CAD build for the part. Positions are in the model's coordinates, mm. A direction names the side the tool comes from. Coordinates: 2 decimals unless noted, no trailing zeros. Loops run counter-clockwise (first coordinate to the right, second up) from the corner with the lowest first, then second, coordinate; pieces in that order, holes last. Notation, with made-up numbers: (18.25, 20.25) -> (38.25, 20.25) arc R9 cw to (38.25, 36.25) -> close; hole circle Ø3 at (-31.75, 19.5). An arc over 180 degrees is marked (long way). Write each question's results on one line, items separated by ' | '.
Autodesk Inventor part; units mm, degrees
ref_plane "YZ Plane" through (0, 0, 0) normal (1, 0, 0) x (0, 1, 0)
ref_plane "XZ Plane" through (0, 0, 0) normal (0, 1, 0) x (-1, 0, 0)
ref_plane "XY Plane" through (0, 0, 0) normal (0, 0, 1) x (1, 0, 0)
sketch "Sketch1" plane through (0, 0, 0) normal (0, 1, 0) x (-1, 0, 0)
  line L0 (0, 44.45) -> (-22.5, 44.45)
  line L1 (-22.5, 44.45) -> (-67.5, 24.15)
  line L2 (-67.5, 24.15) -> (-90, 24.15)
  line L3 (-90, 0) -> (0, 0)
  line L4 (-90, 22.15) -> (-66.3402, 22.15)
  line L5 (-66.3402, 22.15) -> (-22.0052, 42.15)
  line L6 (-22.0052, 42.15) -> (0, 42.15)
  line L7 (-90, 0) -> (-90, 22.15) construction
  line L8 (-90, 24.15) -> (-90, 22.15)
  line L9 (0, 44.45) -> (0, 42.15)
  line L10 (0, 0) -> (0, 42.15) construction
  line L11 (-45, 34.3) -> (-44.0542, 32.2035) construction
  dimension "d0" = 88.9
  dimension "d1" = 48.3
  dimension "d2" = 2.3
  dimension "d3" = 2
  dimension "d4" = 90
  dimension "d5" = 22.5
  dimension "d6" = 22.5
  dimension "d10" = 2.3
revolve "Revolution1" add sketch "Sketch1" angle 360 about axis through (90, 0, 0) along (-1, 0, 0)
equation "\"d0\" = D1"
equation "\"d1\" = D2"
equation "\"d2\" = s1"
equation "\"d3\" = s2"
equation "\"d4\" = L"
equation "\"d5\" = 0.25 * L"
equation "\"d6\" = 0.25 * L"
equation "\"d10\" = s3"
equation "\"s1\" = 2.3"
equation "\"D1\" = 88.9"
equation "\"D2\" = 48.3"
equation "\"L\" = 90"
equation "\"s2\" = 2"
equation "\"s3\" = 2.3"
equation "\"Size_Designation\" = 1.2345"
properties part number "DIN 2616 Concentric Reducer (K) 88.9 x 2.3 - 48.3 x 2" material "Steel"
Q1. Pull direction Z, two halves, no side cores. Call faces 3 (the flat face through (90, -20, 11)), 4 (the cylindrical face through (78.908, -1.062, -24.127)), 5 (the cylindrical face through (78.004, -21.623, -4.802)): +Z half, -Z half, draft (parallel to the pull), parting line (faces both ways), or undercut.
Results are:
face 3: draft | face 4: parting line | face 5: undercut
Q2. Cut at A-A on z = 0. Write the cut outline in (x, y).
Results are:
outline: (0, -44.45) -> (22.5, -44.45) -> (67.5, -24.15) -> (90, -24.15) -> (90, -22.15) -> (66.34, -22.15) -> (22.01, -42.15) -> (0, -42.15) -> close; (0, 42.15) -> (22.01, 42.15) -> (66.34, 22.15) -> (90, 22.15) -> (90, 24.15) -> (67.5, 24.15) -> (22.5, 44.45) -> (0, 44.45) -> close
Q3. Drop flat-ended pins along their axis: pin 1 (12 mm diameter, centred on x = 62, z = -2.5, fed in from +Y); pin 2 (10 mm diameter, centred on x = 44, y = 10.5, fed in from -Z); pin 3 (1.5 mm diameter, centred on y = 20, z = 33, fed in from -X); pin 4 (10 mm diameter, centred on x = 79.5, y = 30, fed in from +Z) (1 decimal). Give the stop position or say it passes through.
Results are:
pin 1: y = 29.26 | pin 2: z = -35.83 | pin 3: x = 28.24 | pin 4: through
Q4. Which spindle directions (+Z, -Z, +X, -X, +Y, -Y) get a long thin tool onto all of the face, cutting with end or side? Do faces 1 (the flat face through (0, -16.3, 39.3)), 2 (the cylindrical face through (10.849, -25.648, -33.449)). Say none if no direction does.
Results are:
face 1: +Z, -Z, -X, +Y, -Y | face 2: -X
Q5. Cut at C-C on x = 10. Write the cut outline in (y, z), and give its area (3 significant figures).
Results are:
outline: circle Ø88.9 at (0, 0); hole circle Ø84.3 at (0, 0) | area: 626 mm^2
Q6. Cut at D-D on x = 45.5. Write the cut outline in (y, z).
Results are:
outline: circle Ø68.15 at (0, 0); hole circle Ø63.1 at (0, 0)
Q7. Wall check: L1, parallel to Y at x = 81, z = 0; L2, parallel to Z at x = 86, y = -4.5; L3, parallel to Z at x = 19, y = 15.5. Give the ranges that are in metal, low to high. Write a range as from..to.
Results are:
L1: -24.15..-22.15, 22.15..24.15 | L2: -23.73..-21.69, 21.69..23.73 | L3: -41.66..-39.2, 39.2..41.66
